from build123d import *

# Parameters (mm, degrees)
SKETCH1_W                = 1200
SKETCH1_H                = 650
BOSS_EXTRUDE1_DEPTH      = 120
SKETCH6_W                = 1075.440948148
SKETCH6_H                = 524.60534056
CUT_EXTRUDE5_DEPTH       = 78
SKETCH2_W                = 100
SKETCH2_H                = 61.240681987
SKETCH2_H_2              = 52.060088527
SKETCH2_H_3              = 44.191008419
BOSS_EXTRUDE3_DEPTH      = 98
SKETCH7_W                = 44.191008419
SKETCH7_H                = 49
CUT_EXTRUDE6_DEPTH       = 91
CUT_EXTRUDE6_DEPTH_BACK  = 1111
SKETCH8_W                = 61.240681987
SKETCH8_H                = 49
CUT_EXTRUDE7_DEPTH       = 91
CUT_EXTRUDE7_DEPTH_BACK  = 1111
SKETCH10_W               = 96.846541068
SKETCH10_H               = 40.58098524
SKETCH10_W_2             = 96.178240502
SKETCH10_H_2             = 36.675881957
SKETCH10_W_3             = 89.939369206
SKETCH10_H_3             = 53.297884326
SKETCH10_W_4             = 93.422548206
SKETCH10_H_4             = 37.665233543
CUT_EXTRUDE9_DEPTH       = 38
SKETCH11_R               = 12.656806897
SKETCH11_R_2             = 13.624607795
SKETCH11_R_3             = 12.31829203
SKETCH11_R_4             = 17.162338859
CUT_EXTRUDE10_DEPTH      = 88
CUT_EXTRUDE10_DEPTH_BACK = 34


with BuildPart() as part:
    # Sketch1 → Boss-Extrude1 (new body)
    with BuildSketch(Plane(origin=(0, 0, 0), x_dir=(1, 0, 0), z_dir=(0, 1, 0))):
        Rectangle(SKETCH1_W, SKETCH1_H)
    extrude(amount=BOSS_EXTRUDE1_DEPTH)

    # Sketch6 → Cut-Extrude5 (cut)
    with BuildSketch(Plane(origin=(0, 120, 0), x_dir=(1, 0, 0), z_dir=(0, 1, 0))):
        Rectangle(SKETCH6_W, SKETCH6_H)
    extrude(amount=-CUT_EXTRUDE5_DEPTH, mode=Mode.SUBTRACT)

    # Sketch2 → Boss-Extrude3 (add)
    with BuildSketch(Plane(origin=(0, 120, 0), x_dir=(1, 0, 0), z_dir=(0, 1, 0))):
        with Locations((460, 355.620340994)):
            Rectangle(SKETCH2_W, SKETCH2_H)
        with Locations((-460, 351.030044264)):
            Rectangle(SKETCH2_W, SKETCH2_H_2)
        with Locations((-460, -347.09550421)):
            Rectangle(SKETCH2_W, SKETCH2_H_3)
        with Locations((460, -347.09550421)):
            Rectangle(SKETCH2_W, SKETCH2_H_3)
    extrude(amount=-BOSS_EXTRUDE3_DEPTH)

    # Sketch7 → Cut-Extrude6 (cut, two sides)
    with BuildSketch(Plane(origin=(510, 0, 0), x_dir=(0, 0, -1), z_dir=(1, 0, 0))) as cut_extrude6_sk:
        with Locations((-347.09550421, 95.5)):
            Rectangle(SKETCH7_W, SKETCH7_H)
    extrude(amount=CUT_EXTRUDE6_DEPTH, mode=Mode.SUBTRACT)
    extrude(cut_extrude6_sk.sketch, amount=-CUT_EXTRUDE6_DEPTH_BACK, mode=Mode.SUBTRACT)

    # Sketch8 → Cut-Extrude7 (cut, two sides)
    with BuildSketch(Plane(origin=(510, 0, 0), x_dir=(0, 0, -1), z_dir=(1, 0, 0))) as cut_extrude7_sk:
        with Locations((355.620340994, 95.5)):
            Rectangle(SKETCH8_W, SKETCH8_H)
    extrude(amount=CUT_EXTRUDE7_DEPTH, mode=Mode.SUBTRACT)
    extrude(cut_extrude7_sk.sketch, amount=-CUT_EXTRUDE7_DEPTH_BACK, mode=Mode.SUBTRACT)

    # Sketch10 → Cut-Extrude9 (cut)
    with BuildSketch(Plane(origin=(0, 71, 0), x_dir=(1, 0, 0), z_dir=(0, 1, 0))):
        with Locations((-460, -347.095504209)):
            Rectangle(SKETCH10_W, SKETCH10_H)
        with Locations((460, -347.09550421)):
            Rectangle(SKETCH10_W_2, SKETCH10_H_2)
        with Locations((460, 355.620340993)):
            Rectangle(SKETCH10_W_3, SKETCH10_H_3)
        with Locations((-460, 355.620340994)):
            Rectangle(SKETCH10_W_4, SKETCH10_H_4)
    extrude(amount=-CUT_EXTRUDE9_DEPTH, mode=Mode.SUBTRACT)

    # Sketch11 → Cut-Extrude10 (cut, two sides)
    with BuildSketch(Plane(origin=(0, 33, 0), x_dir=(1, 0, 0), z_dir=(0, 1, 0))) as cut_extrude10_sk:
        with Locations((-462.307183801, 358.120386365)):
            Circle(SKETCH11_R)
        with Locations((-462.307183801, -349.182945784)):
            Circle(SKETCH11_R_2)
        with Locations((463.409280552, -349.182945784)):
            Circle(SKETCH11_R_3)
        with Locations((467.367852557, 358.120386365)):
            Circle(SKETCH11_R_4)
    extrude(amount=CUT_EXTRUDE10_DEPTH, mode=Mode.SUBTRACT)
    extrude(cut_extrude10_sk.sketch, amount=-CUT_EXTRUDE10_DEPTH_BACK, mode=Mode.SUBTRACT)


solid = part.part
Source: CAD feature listing. Evaluate the final solid. Frame: model axes, mm. A direction names the side the tool comes from. Give positions to 0.01 mm unless a question says otherwise; leave off trailing zeros. Write each loop counter-clockwise with the first axis right and the second up, starting at its lowest first coordinate (ties: lowest second). Pieces come first, ordered by that corner, then holes. Notation, with made-up numbers: M 56.5,38.5 L 60.5,38.5 A16 ccw 60.5,49.5 Z; hole C 6.25,-31 d4. An arc over 180 degrees is marked long. Answer as a JSON object with one key per item and string values.
Q1. Mould query, pull axis Z, two halves, no side actions, for faces 1 (the face through (-8, 42, -4)), 2 (the face through (-461, 47, 369.191)), 3 (the face through (-47, 120, 263)). Classes: +Z half, -Z half, draft (parallel to the pull), parting line (faces both ways), or undercut.
Geometry check:
{"face 1": "undercut", "face 2": "+Z half", "face 3": "draft"}
Q2. Contact query for flat-ended pins moving along their axis: P1, Ø19, axis at y = 47.5, z = -345.5, coming from the +X side; P2, Ø8, axis at x = 155.5, y = 107, coming from the +Z side; P3, Ø22, axis at x = 444, z = 338, coming from the -Y side. Output: stop coordinate, or through.
Geometry check:
{"P1": "stops at x = 510", "P2": "stops at z = 325", "P3": "stops at y = 22"}
Q3. Ray query, line 1 along Z through (x, y) = (-447, 43.5); line 2 along X through (y, z) = (43, -331.5); line 3 along Z through (x, y) = (-257, 83). Return the intervals inside material, ascending.
Geometry check:
{"line 1": "z = -377.06 to -374.45, -336.79 to -262.3, 262.3 to 326.81, 367.39 to 369.19", "line 2": "x = -510 to -410, 410 to 415.03, 504.97 to 510", "line 3": "z = -325 to -262.3, 262.3 to 325"}
Q4. Cut plane C-C, the plane x = 316.5. Return the cut outline in (y, z), then the cut area to 3 significant figures.
Geometry check:
{"outline": "M 0,-325 L 120,-325 L 120,-262.3 L 42,-262.3 L 42,262.3 L 120,262.3 L 120,325 L 0,325 Z", "area": "37,100 mm^2"}
Q5. Cut plane B-B, the plane z = -4. Return the cut outline in (x, y).
Geometry check:
{"outline": "M -600,0 L 600,0 L 600,120 L 537.72,120 L 537.72,42 L -537.72,42 L -537.72,120 L -600,120 Z"}
Q6. Cut plane A-A, the plane y = 88.5. Return the cut outline in (x, z), then the cut area to 3 significant figures.
Geometry check:
{"outline": "M -600,-325 L 600,-325 L 600,325 L -600,325 Z; hole M -537.72,-262.3 L 537.72,-262.3 L 537.72,262.3 L -537.72,262.3 Z", "area": "216,000 mm^2"}
Q7. Access query for faces 4 (the face through (-460, 71, 326)), 5 (the face through (-450, 22, 342)), 6 (the face through (459, 52, 328.758)), 7 (the face through (-8, 0, -5)), 8 (the face through (510, 47, -355)). Directions: +Z, -Z, +X, -X, +Y, -Y. A direction counts if a zero-diameter tool reaches every point of the face in a straight line with its end or side. Return the directions, or none.
Geometry check:
{"face 4": "+Z, +X, -X, +Y", "face 5": "+Z, +X, -X, -Y", "face 6": "+Y", "face 7": "+Z, -Z, +X, -X, -Y", "face 8": "-Z, +X, +Y, -Y"}
